Could you check a few things on this model? Use its own coordinates, in mm. Round coordinates to 2 decimals unless told otherwise and drop trailing zeros. Loops run counter-clockwise (first coordinate to the right, second up) from the corner with the lowest first, then second, coordinate; pieces in that order, holes last. Notation, with made-up numbers: (88.25, 30.5) - (123.25, 30.5) arc R13 cw to (123.25, 37.5) - close; hole circle Ø5 at (-1, 5). An arc over 180 degrees is marked (long way). Use one line per item in the form item = value.
```python
from build123d import *

# Parameters (mm, degrees)
SKETCH1_R           = 10
BOSS_EXTRUDE1_DEPTH = 1
SKETCH2_R           = 10
CUT_EXTRUDE1_DEPTH  = 1
SKETCH3_R           = 20
CUT_EXTRUDE2_DEPTH  = 1
CUT_EXTRUDE3_DEPTH  = 127.23292637
BOSS_EXTRUDE2_DEPTH = 1
BOSS_EXTRUDE4_DEPTH = 1


with BuildPart() as part:
    # Sketch1 → Boss-Extrude1 (new body)
    with BuildSketch(Plane.XY):
        with BuildLine():
            Line((94.42701916, 40.188914375), (53.885, 40))
            Line((53.885, 40), (-53.885, 40))
            Line((-53.885, 40), (-53.885, -40))
            Line((-53.885, -40), (53.885, -40))
            ThreePointArc((53.885, -40), (85.857258243, -25.182373866), (112.594107484, -2.227456438))
            ThreePointArc((112.594107484, -2.227456438), (117.686467499, 24.925594205), (94.66, 40.19))
            Line((94.66, 40.19), (94.42701916, 40.188914375))
        make_face()
        with Locations((91.76, 19.26)):
            Circle(SKETCH1_R, mode=Mode.SUBTRACT)
    extrude(amount=BOSS_EXTRUDE1_DEPTH)

    # Sketch2 → Cut-Extrude1 (cut)
    with BuildSketch(Plane.XY.offset(1)):
        Circle(SKETCH2_R)
    extrude(amount=-CUT_EXTRUDE1_DEPTH, mode=Mode.SUBTRACT)

    # Sketch3 → Cut-Extrude2 (cut)
    with BuildSketch(Plane.XY.offset(1)):
        with Locations((94.66, 15.19)):
            Circle(SKETCH3_R)
    extrude(amount=-CUT_EXTRUDE2_DEPTH, mode=Mode.SUBTRACT)

    # Sketch4 → Cut-Extrude3 (cut, through all)
    with BuildSketch(Plane.XY.offset(1)):
        with BuildLine():
            Line((-53.885, 40), (-30, 40))
            ThreePointArc((-30, 40), (-50, 0), (-30, -40))
            Line((-30, -40), (-53.885, -40))
            Line((-53.885, -40), (-53.885, 40))
        make_face()
    extrude(amount=-CUT_EXTRUDE3_DEPTH, mode=Mode.SUBTRACT)

    # Sketch5 → Boss-Extrude2 (add)
    with BuildSketch(Plane.XY.offset(1)):
        with BuildLine():
            Line((-30, -40), (30, -40))
            ThreePointArc((30, -40), (0, -50), (-30, -40))
        make_face()
    extrude(amount=-BOSS_EXTRUDE2_DEPTH)

    # Sketch6 → Boss-Extrude4 (add)
    with BuildSketch(Plane.XY.offset(1)):
        with BuildLine():
            Line((-30, 40), (-30, 147))
            ThreePointArc((-30, 147), (-29.121320344, 149.121320344), (-27, 150))
            Line((-27, 150), (27, 150))
            ThreePointArc((27, 150), (29.121320344, 149.121320344), (30, 147))
            Line((30, 147), (30, 40))
            Line((30, 40), (-30, 40))
        make_face()
        Polygon((-1, 128), (-1, 112), (-10, 112), (-10, 110), (10, 110), (10, 112), (1, 112), (1, 128), (10, 128), (10, 130), (-10, 130), (-10, 128), align=None, mode=Mode.SUBTRACT)
    extrude(amount=-BOSS_EXTRUDE4_DEPTH)


solid = part.part
```
1. We'd pull the mould along Y, two halves only. Please class faces 1 (the face through (79.92, 28.71, 0.51)), 2 (the face through (17, 29, 0)), 3 (the face through (117.84, 24.55, 0.49)): +Y half, -Y half, draft (parallel to the pull), parting line (faces both ways), or undercut.
Solution:
face_1 = undercut
face_2 = draft
face_3 = parting line
2. If we section it at A-A, the plane z = 0.15: Write out the boundary of the cut face in (x, y) (3 decimals), plus the area to 3 significant figures.
Solution:
outline = (-30, 40) arc R50 ccw to (30, -40) - (53.885, -40) arc R128.337 ccw to (112.594, -2.227) arc R25 ccw to (94.66, 40.19) - (53.885, 40) - (30, 40) - (30, 147) arc R3 ccw to (27, 150) - (-27, 150) arc R3 ccw to (-30, 147) - close; hole circle Ø20 at (0, 0); hole (-10, 110) - (10, 110) - (10, 112) - (1, 112) - (1, 128) - (10, 128) - (10, 130) - (-10, 130) - (-10, 128) - (-1, 128) - (-1, 112) - (-10, 112) - close; hole circle Ø40 at (94.66, 15.19)
area = 17,100 mm^2
3. If we section it at B-B, the plane x = 97.5: Write out the boundary of the cut face in (y, z).
Solution:
outline = (-16.73, 0) - (-4.61, 0) - (-4.61, 1) - (-16.73, 1) - close; (34.99, 0) - (40.03, 0) - (40.03, 1) - (34.99, 1) - close
4. If we section it at D-D, the plane x = -7: Write out the boundary of the cut face in (y, z).
Solution:
outline = (-49.51, 0) - (-7.14, 0) - (-7.14, 1) - (-49.51, 1) - close; (7.14, 0) - (110, 0) - (110, 1) - (7.14, 1) - close; (112, 0) - (128, 0) - (128, 1) - (112, 1) - close; (130, 0) - (150, 0) - (150, 1) - (130, 1) - close
5. Please list where these lines run through material, in increasing order: line 1 along Y through (x, z) = (0, 0.7); line 2 along X through (y, z) = (123.5, 0.35); line 3 along Y through (x, z) = (6.5, 0.65).
Solution:
line_1 = -50 to -10, 10 to 110, 130 to 150
line_2 = -30 to -1, 1 to 30
line_3 = -49.58 to -7.6, 7.6 to 110, 112 to 128, 130 to 150
6. For P1, Ø0.5, axis at y = 111, z = 0.5, coming from the -X side; P2, Ø0.5, axis at y = 123.5, z = 0.5, coming from the +X side; P3, Ø0.5, axis at x = 45.5, z = 0.5, coming from the -Y side, each with a flat end and sliding along its axis, tell me the tip position at first contact or that it passes through.
Solution:
P1 = -30
P2 = 30
P3 = -40
7. If we section it at C-C, the plane y = 15.19: Write out the boundary of the cut face in (x, z).
Solution:
outline = (-47.64, 0) - (74.66, 0) - (74.66, 1) - (-47.64, 1) - close; (114.66, 0) - (119.66, 0) - (119.66, 1) - (114.66, 1) - close
